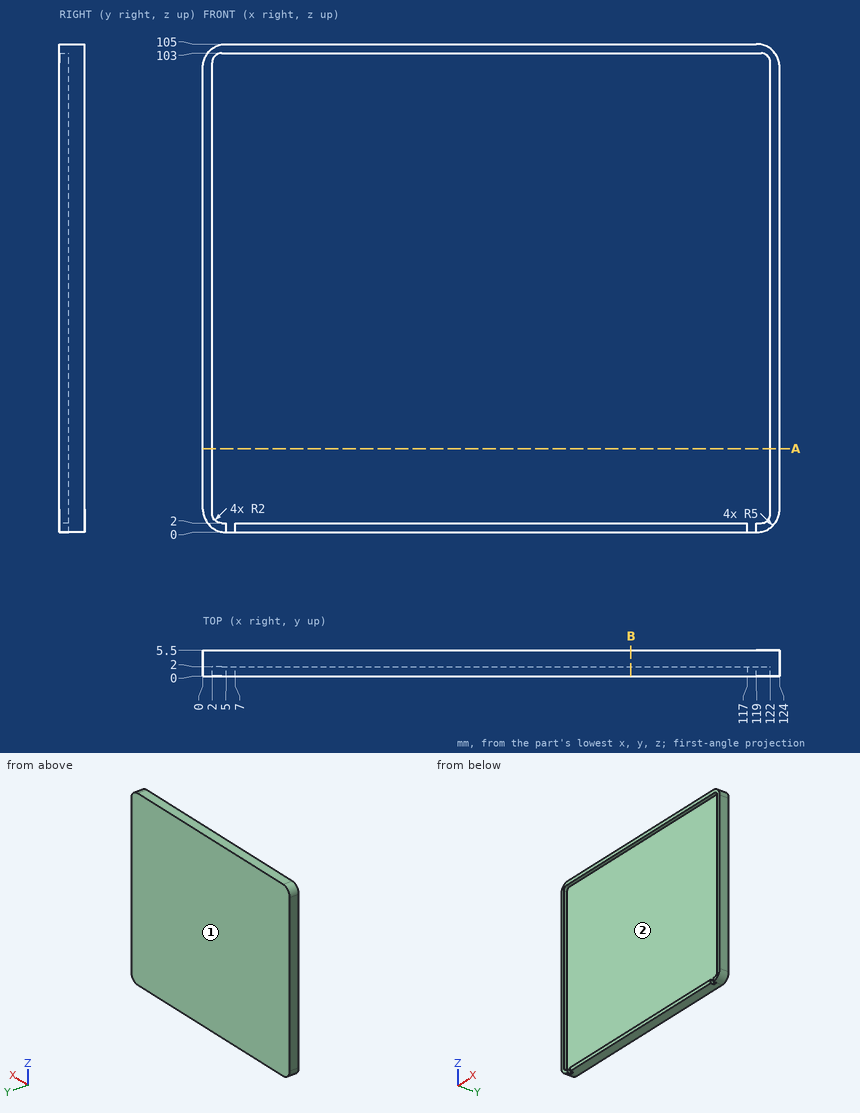
Check sheet for the drawn part. Datum: minimum x, y, z corner. Units: mm. Round coordinates to 2 decimals unless told otherwise and drop trailing zeros. Write each loop counter-clockwise with the first axis right and the second up, starting at its lowest first coordinate (ties: lowest second). Pieces come first, ordered by that corner, then holes. Notation, with made-up numbers: (-2, 41.25) - (4, 41.25) arc R24 cw to (4, 55.25) - close; hole circle Ø7 at (-40, -30.75). An arc over 180 degrees is marked (long way). Return JSON: item names as keys, results as strings.
Q1. Cross-section at A-A (z = 18). Record the boundary of the cut face in (x, y), then the cut area to 3 significant figures.
Returned:
{"outline": "(0, 0) - (2, 0) - (2, 2) - (122, 2) - (122, 0) - (124, 0) - (124, 5.5) - (0, 5.5) - close", "area": "442 mm²"}
Q2. Draft check along Z on the marked faces 1 and 2. Enter one of: released by +Z, released by -Z, zero draft, split by the parting line, or undercut.
Returned:
{"face 1": "zero draft", "face 2": "undercut"}
Q3. Depth check by flat-ended pin: P1, Ø1.5, axis at x = 18, z = 64.5, coming from the -Y side; P2, Ø0.6, axis at y = 1, z = 1.5, coming from the +X side; P3, Ø1.6, axis at y = 0.5, z = 1, coming from the -X side. Enter the tip coordinate at first touch or a pass-through.
Returned:
{"P1": "stops at y = 2", "P2": "stops at x = 122.84", "P3": "stops at x = 1.16"}
Q4. Cross-section at B-B (x = 92). Record the boundary of the cut face in (y, z), then the cut area to 4 significant figures.
Returned:
{"outline": "(0, 0) - (5.5, 0) - (5.5, 105) - (0, 105) - (0, 103) - (2, 103) - (2, 2) - (0, 2) - close", "area": "375.5 mm²"}
Q5. Scan lines: L1, parallel to Z at x = 96, y = 1.45; L2, parallel to X at y = 1.15, z = 39; L3, parallel to Y at x = 71, z = 100. Record each from-to range of solid material in increasing order. Write a range as from..to.
Returned:
{"L1": "z = 0..2, 103..105", "L2": "x = 0..2, 122..124", "L3": "y = 2..5.5"}
